from build123d import *

# Parameters (mm, degrees)
SKETCH1_R           = 3
BOSS_EXTRUDE1_DEPTH = 13
SKETCH2_R           = 1
CUT_EXTRUDE1_DEPTH  = 13
CUT_EXTRUDE2_DEPTH  = 12


with BuildPart() as part:
    # Sketch1 → Boss-Extrude1 (new body)
    with BuildSketch(Plane(origin=(0, 0, 0), x_dir=(1, 0, 0), z_dir=(0, 1, 0))):
        with Locations(Location((0, 0, 0), (0, 0, 90))):
            Circle(SKETCH1_R)
    extrude(amount=BOSS_EXTRUDE1_DEPTH)

    # Sketch2 → Cut-Extrude1 (cut)
    with BuildSketch(Plane(origin=(0, 13, 0), x_dir=(1, 0, 0), z_dir=(0, 1, 0))):
        with Locations(Location((0, 0, 0), (0, 0, 270))):
            Circle(SKETCH2_R)
    extrude(amount=-CUT_EXTRUDE1_DEPTH, mode=Mode.SUBTRACT)

    # Sketch3 → Cut-Extrude2 (cut)
    with BuildSketch(Plane(origin=(0, 13, 0), x_dir=(1, 0, 0), z_dir=(0, 1, 0))):
        Polygon((26.073564647, -2.5), (1.658312395, -2.5), (-1.658312395, -2.5), (-26.073564647, -2.5), (-26.073564647, -51.330504504), (26.073564647, -51.330504504), align=None)
    extrude(amount=-CUT_EXTRUDE2_DEPTH, mode=Mode.SUBTRACT)


solid = part.part
Check sheet for the modelled part. Datum: model origin and axes. Units: mm. Coordinates: 2 decimals unless noted, no trailing zeros. Loops run counter-clockwise (first coordinate to the right, second up) from the corner with the lowest first, then second, coordinate; pieces in that order, holes last. Notation, with made-up numbers: (80, 64.25) -> (134, 64.25) arc R32 cw to (134, 100.25) -> close; hole circle Ø4 at (57, -23.75). An arc over 180 degrees is marked (long way). Answer in a Markdown table with one row per item.
1. Material ranges on line 1 along X through (y, z) = (6.5, 0); line 2 along Z through (x, y) = (0.9, 3.25); line 3 along X through (y, z) = (3.75, -0.8), recorded low to high. Write a range as [from, to].
Check values:
| item | result |
|---|---|
| line 1 | x = [-3, -1], [1, 3] |
| line 2 | z = [-2.86, -0.44], [0.44, 2.5] |
| line 3 | x = [-2.89, -0.6], [0.6, 2.89] |
2. Sectioned sample at B-B, the plane x = 0. Record the boundary of the cut face in (y, z), then the cut area to 3 significant figures.
Check values:
| item | result |
|---|---|
| outline | (0, -3) -> (13, -3) -> (13, -1) -> (0, -1) -> close; (0, 1) -> (13, 1) -> (13, 2.5) -> (1, 2.5) -> (1, 3) -> (0, 3) -> close |
| area | 46.0 mm2 |
3. Sectioned sample at A-A, the plane z = 0. Record the boundary of the cut face in (x, y).
Check values:
| item | result |
|---|---|
| outline | (-3, 0) -> (-1, 0) -> (-1, 13) -> (-3, 13) -> close; (1, 0) -> (3, 0) -> (3, 13) -> (1, 13) -> close |
4. Go/stop test with flat-tipped pins: pin 1 (1 mm diameter, centred on x = 0.5, y = 7, fed in from +Z); pin 2 (1 mm diameter, centred on y = 4, z = -2.5, fed in from -X); pin 3 (1.8 mm diameter, centred on x = 0, z = 0, fed in from -Y). Record where each tip stops, or that it passes through.
Check values:
| item | result |
|---|---|
| pin 1 | stops at z = 2.5 |
| pin 2 | stops at x = -2.24 |
| pin 3 | passes through |
5. Release check for a two-part mould opening along Z. For faces 1 (the face through (-1, 0, 1)), 2 (the face through (0, 7, 2.5)), 3 (the face through (-1, 7, 0)) record: released by +Z, released by -Z, zero draft, split by the parting line, or undercut.
Check values:
| item | result |
|---|---|
| face 1 | zero draft |
| face 2 | released by +Z |
| face 3 | undercut |
6. Sectioned sample at C-C, the plane y = 5.5. Record the boundary of the cut face in (x, z).
Check values:
| item | result |
|---|---|
| outline | (-1.66, 2.5) arc R3 ccw (long way) to (1.66, 2.5) -> close; hole circle Ø2 at (0, 0) |
7. Sectioned sample at D-D, the plane x = -2.6. Record the boundary of the cut face in (y, z), then the cut area to 3 significant figures.
Check values:
| item | result |
|---|---|
| outline | (0, -1.5) -> (13, -1.5) -> (13, 1.5) -> (0, 1.5) -> close |
| area | 38.9 mm2 |
